Read the model definition and answer for the solid it produces. Units are mm, in the model's axes. A direction names the side the tool comes from. Coordinates: 2 decimals unless noted, no trailing zeros. Order: outer loops, then holes, each group sorted by start corner. A loop starts at its lowest first (then second) coordinate and runs counter-clockwise, first axis right, second up.
```python
from build123d import *

# Parameters (mm, degrees)
SKETCH1_R              = 4.85
SKETCH1_R_2            = 3
SKETCH1_R_3            = 2.15
BOSS_EXTRUDE1_DEPTH    = 27.5
BOSS_EXTRUDE2_START    = -2.8
SKETCH1_3_R            = 6.5
SKETCH1_3_R_2          = 4.85
SKETCH1_3_R_3          = 3
SKETCH1_3_R_4          = 2.15
BOSS_EXTRUDE2_DEPTH    = 2.8
CUT_EXTRUDE1_START     = 22
CUT_EXTRUDE1_OUTLINE_R = 2.15
CUT_EXTRUDE1_DEPTH     = 3
CUT_EXTRUDE2_START     = 12.5
SKETCH2_3_R            = 2.15
CUT_EXTRUDE2_DEPTH     = 15
CUT_EXTRUDE3_START     = 22
CUT_EXTRUDE3_DEPTH     = 15
CUT_EXTRUDE4_START     = -2.8
SKETCH3_R              = 2.35
CUT_EXTRUDE4_DEPTH     = 1


# Read off the part's stored shape, not the designer's step: Cut-Extrude1
with BuildPart() as part:
    # Sketch1 → Boss-Extrude1 (new body)
    # profile 1 of 3: a face of its own
    with BuildSketch(Plane(origin=(0, 0, 0), x_dir=(1, 0, 0), z_dir=(0, 1, 0))):
        with Locations(Location((0, 0, 0), (0, 0, 270))):
            Circle(SKETCH1_R)
        Circle(SKETCH1_R_2, mode=Mode.SUBTRACT)
    # profile 2 of 3: a face of its own
    with BuildSketch(Plane(origin=(0, 0, 0), x_dir=(1, 0, 0), z_dir=(0, 1, 0))):
        Circle(SKETCH1_R_2)
        Circle(SKETCH1_R_3, mode=Mode.SUBTRACT)
    # profile 3 of 3: a face of its own
    with BuildSketch(Plane(origin=(0, 0, 0), x_dir=(1, 0, 0), z_dir=(0, 1, 0))):
        Circle(SKETCH1_R_3)
    extrude(amount=BOSS_EXTRUDE1_DEPTH)

    # Sketch1<3> → Boss-Extrude2 (add)
    # profile 1 of 4: a face of its own
    with BuildSketch(Plane(origin=(0, 0, 0), x_dir=(1, 0, 0), z_dir=(0, 1, 0)).offset(BOSS_EXTRUDE2_START)):
        with Locations(Location((0, 0, 0), (0, 0, 270))):
            Circle(SKETCH1_3_R)
        with Locations(Location((0, 0, 0), (0, 0, 270))):
            Circle(SKETCH1_3_R_2, mode=Mode.SUBTRACT)
    # profile 2 of 4: a face of its own
    with BuildSketch(Plane(origin=(0, 0, 0), x_dir=(1, 0, 0), z_dir=(0, 1, 0)).offset(BOSS_EXTRUDE2_START)):
        with Locations(Location((0, 0, 0), (0, 0, 270))):
            Circle(SKETCH1_3_R_2)
        Circle(SKETCH1_3_R_3, mode=Mode.SUBTRACT)
    # profile 3 of 4: a face of its own
    with BuildSketch(Plane(origin=(0, 0, 0), x_dir=(1, 0, 0), z_dir=(0, 1, 0)).offset(BOSS_EXTRUDE2_START)):
        Circle(SKETCH1_3_R_3)
        Circle(SKETCH1_3_R_4, mode=Mode.SUBTRACT)
    # profile 4 of 4: a face of its own
    with BuildSketch(Plane(origin=(0, 0, 0), x_dir=(1, 0, 0), z_dir=(0, 1, 0)).offset(BOSS_EXTRUDE2_START)):
        Circle(SKETCH1_3_R_4)
    extrude(amount=BOSS_EXTRUDE2_DEPTH)

    # Cut-Extrude1 outline → Cut-Extrude1 (cut)
    with BuildSketch(Plane(origin=(0, 0, 0), x_dir=(1, 0, 0), z_dir=(0, 1, 0)).offset(CUT_EXTRUDE1_START)):
        with BuildLine():
            ThreePointArc((-3.135681744, 3.7), (-4.85, 0), (-3.135681744, -3.7))
            Line((-3.135681744, -3.7), (3.135681744, -3.7))
            ThreePointArc((3.135681744, -3.7), (4.85, 0), (3.135681744, 3.7))
            Line((3.135681744, 3.7), (-3.135681744, 3.7))
        make_face()
        Circle(CUT_EXTRUDE1_OUTLINE_R, mode=Mode.SUBTRACT)
    extrude(amount=CUT_EXTRUDE1_DEPTH, mode=Mode.SUBTRACT)

    # Sketch2<3> → Cut-Extrude2 (cut)
    with BuildSketch(Plane(origin=(0, 0, 0), x_dir=(1, 0, 0), z_dir=(0, 1, 0)).offset(CUT_EXTRUDE2_START)):
        with Locations(Location((0, 0, 0), (0, 0, 270))):
            Circle(SKETCH2_3_R)
    extrude(amount=CUT_EXTRUDE2_DEPTH, mode=Mode.SUBTRACT)

    # Sketch2<4> → Cut-Extrude3 (cut)
    with BuildSketch(Plane(origin=(0, 0, 0), x_dir=(1, 0, 0), z_dir=(0, 1, 0)).offset(CUT_EXTRUDE3_START)):
        Polygon((4.272391992, 0), (3.135681744, 1.968839903), (3.135681744, -1.968839903), align=None)
        with BuildLine():
            ThreePointArc((4.85, 0), (4.400599758, 2.038926622), (3.135681744, 3.7))
            Line((3.135681744, 3.7), (3.135681744, 1.968839903))
            Line((3.135681744, 1.968839903), (4.272391992, 0))
            Line((4.272391992, 0), (3.135681744, -1.968839903))
            Line((3.135681744, -1.968839903), (3.135681744, -3.7))
            ThreePointArc((3.135681744, -3.7), (4.400599758, -2.038926622), (4.85, 0))
        make_face()
    extrude(amount=CUT_EXTRUDE3_DEPTH, mode=Mode.SUBTRACT)

    # Sketch3 → Cut-Extrude4 (cut)
    with BuildSketch(Plane(origin=(0, 0, 0), x_dir=(1, 0, 0), z_dir=(0, 1, 0)).offset(CUT_EXTRUDE4_START)):
        with Locations(Location((0, 0, 0), (0, 0, 270))):
            Circle(SKETCH3_R)
    extrude(amount=CUT_EXTRUDE4_DEPTH, mode=Mode.SUBTRACT)


solid = part.part
```
1) A cutting plane is placed at D-D, the plane x = 0. Determine the outline of the cut face in (y, z), and give its area (3 significant figures).
A:
outline: (-2.8, -6.5) - (0, -6.5) - (0, -4.85) - (27.5, -4.85) - (27.5, -2.15) - (25, -2.15) - (25, -3.7) - (22, -3.7) - (22, -2.15) - (12.5, -2.15) - (12.5, 2.15) - (22, 2.15) - (22, 3.7) - (25, 3.7) - (25, 2.15) - (27.5, 2.15) - (27.5, 4.85) - (0, 4.85) - (0, 6.5) - (-2.8, 6.5) - (-2.8, 2.35) - (-1.8, 2.35) - (-1.8, -2.35) - (-2.8, -2.35) - close
area: 225 mm2
2) A cutting plane is placed at B-B, the plane x = -4. Determine the outline of the cut face in (y, z).
A:
outline: (-2.8, -5.12) - (0, -5.12) - (0, -2.74) - (22, -2.74) - (22, 2.74) - (0, 2.74) - (0, 5.12) - (-2.8, 5.12) - close; (25, -2.74) - (27.5, -2.74) - (27.5, 2.74) - (25, 2.74) - close
3) Determine the mould class of faces 4 (the flat face through (3.136, 26, 0)), 5 (the cylindrical face through (0.65, 17.18, 2.05)), 6 (the cylindrical face through (-4.735, 13.558, -1.051)) for opening direction X: pulls with the +X half, pulls with the -X half, needs draft (parallel to the pull), parting line crosses it, or undercut.
A:
face 4: pulls with the +X half
face 5: undercut
face 6: parting line crosses it
4) A cutting plane is placed at C-C, the plane y = 18. Determine the outline of the cut face in (x, z).
A:
outline: circle Ø9.7 at (0, 0); hole circle Ø4.3 at (0, 0)
5) Flat-ended cylindrical pins translate along their axes: pin 1 Ø1.2 at (y, z) = (27, 0) entering from +X; pin 2 Ø1.5 at (x, y) = (-2, 9) entering from +Z; pin 3 Ø3 at (x, y) = (2, 7.5) entering from +Z. Find the tip coordinate at first contact, or state that the pin passes through.
A:
pin 1: stops at x = 3.14
pin 2: stops at z = 4.69
pin 3: stops at z = 4.82
6) Straight lines are drawn through the part: line 1 (X direction, y = -2.2, z = 0); line 2 (X direction, y = 26.6, z = 0); line 3 (Y direction, x = 2.25, z = 0.25). For each, find the intervals that lie inside material, in ascending order.
A:
line 1: x = -6.5 to -2.35, 2.35 to 6.5
line 2: x = -4.85 to -2.15, 2.15 to 3.14
line 3: y = -1.8 to 22, 25 to 27.5
7) A cutting plane is placed at A-A, the plane z = 0. Determine the outline of the cut face in (x, y), and give its area (3 significant figures).
A:
outline: (-6.5, -2.8) - (-2.35, -2.8) - (-2.35, -1.8) - (2.35, -1.8) - (2.35, -2.8) - (6.5, -2.8) - (6.5, 0) - (4.85, 0) - (4.85, 22) - (2.15, 22) - (2.15, 12.5) - (-2.15, 12.5) - (-2.15, 22) - (-4.85, 22) - (-4.85, 0) - (-6.5, 0) - close; (-4.85, 25) - (-2.15, 25) - (-2.15, 27.5) - (-4.85, 27.5) - close; (2.15, 25) - (3.14, 25) - (3.14, 27.5) - (2.15, 27.5) - close
area: 213 mm2
8) Which of the six approach directions +Z, -Z, +X, -X, +Y, -Y give full straight-line access (tool end or side, diameter ignored) to faces 1 (the flat face through (0, 12.5, 0)), 2 (the flat face through (0, 23, 3.7)), 3 (the cylindrical face through (0.71, -2.31, 2.24))?
A:
face 1: +Y
face 2: +X, -X
face 3: -Y
